from build123d import *

# Parameters (mm, degrees)
F0_W          = 20
F0_H          = 26
F1_DEPTH      = 28
F3_DEPTH      = 3.25
F3_DEPTH_BACK = 3.25
F4_T1_DEPTH   = 6.3508529611
F4_T3_DEPTH   = 6.3508529611
F4_T5_DEPTH   = 6.3508529611
F4_T7_DEPTH   = 6.3508529611
F4_T9_DEPTH   = 51.7168298797
F4_T11_DEPTH  = 45.7168298797
F4_T13_DEPTH  = 53.7168298797
F4_T15_DEPTH  = 32.4668298797
F4_T17_DEPTH  = 32.4668298797


# Not quite as in the source:
# - a fillet or chamfer that OpenCascade refuses, or shapes differently, is made with other operations: its cross-section is extruded or revolved along the edge and cut away or added


with BuildPart() as f1:
    # F0 (on Top) → F1 (new body)
    with BuildSketch(Plane.XY):
        Rectangle(F0_W, F0_H)
    extrude(amount=F1_DEPTH)

    # F2 (on Right) → F3 (cut, two sides)
    with BuildSketch(Plane.YZ) as f3_sk:
        Polygon((13, 28), (-11, 28), (-11, 19.4068542495), (-5.3431457505, 13.75), (13, 13.75), align=None)
    extrude(amount=-F3_DEPTH, mode=Mode.SUBTRACT)
    extrude(f3_sk.sketch, amount=F3_DEPTH_BACK, mode=Mode.SUBTRACT)

    # F4: chamfer of 5 on 9 edges, made by hand

    # F4_s2 → F4_t1 (cut)
    with BuildSketch(Plane(origin=(13.6666666667, -13.6666666667, 13.6666666667), x_dir=(0.7071067812, 0.7071067812, 0), z_dir=(0.5773502692, -0.5773502692, 0.5773502692))):
        Polygon((1.4142135624, 11.430952133), (-5.6568542495, 11.430952133), (-2.1213203436, 17.5546764899), align=None)
    extrude(amount=F4_T1_DEPTH, mode=Mode.SUBTRACT)

    # F4_s4 → F4_t3 (cut)
    with BuildSketch(Plane(origin=(13.6666666667, 13.6666666667, 13.6666666667), x_dir=(-0.7071067812, 0.7071067812, 0), z_dir=(0.5773502692, 0.5773502692, 0.5773502692))):
        Polygon((-1.4142135624, 11.430952133), (5.6568542495, 11.430952133), (2.1213203436, 17.5546764899), align=None)
    extrude(amount=F4_T3_DEPTH, mode=Mode.SUBTRACT)

    # F4_s6 → F4_t5 (cut)
    with BuildSketch(Plane(origin=(-13.6666666667, -13.6666666667, 13.6666666667), x_dir=(0.7071067812, -0.7071067812, 0), z_dir=(-0.5773502692, -0.5773502692, 0.5773502692))):
        Polygon((5.6568542495, 11.430952133), (2.1213203436, 17.5546764899), (-1.4142135624, 11.430952133), align=None)
    extrude(amount=F4_T5_DEPTH, mode=Mode.SUBTRACT)

    # F4_s8 → F4_t7 (cut)
    with BuildSketch(Plane(origin=(-13.6666666667, 13.6666666667, 13.6666666667), x_dir=(-0.7071067812, -0.7071067812, 0), z_dir=(-0.5773502692, 0.5773502692, 0.5773502692))):
        Polygon((-5.6568542495, 11.430952133), (-2.1213203436, 17.5546764899), (1.4142135624, 11.430952133), align=None)
    extrude(amount=F4_T7_DEPTH, mode=Mode.SUBTRACT)

    # F4_s10 → F4_t9 (cut)
    with BuildSketch(Plane.XZ.offset(-25.8584149398)):
        Polygon((10, 23), (5, 28), (10, 28), align=None)
        Polygon((-5, 28), (-10, 23), (-10, 28), align=None)
    extrude(amount=F4_T9_DEPTH, mode=Mode.SUBTRACT)

    # F4_s12 → F4_t11 (cut)
    with BuildSketch(Plane.YZ.offset(-22.8584149398)):
        Polygon((-13, 23), (-8, 28), (-13, 28), align=None)
    extrude(amount=F4_T11_DEPTH, mode=Mode.SUBTRACT)

    # F4_s14 → F4_t13 (cut)
    with BuildSketch(Plane.XY.offset(-12.8584149398)):
        Polygon((10, -8), (5, -13), (10, -13), align=None)
        Polygon((-5, -13), (-10, -8), (-10, -13), align=None)
        Polygon((10, 8), (5, 13), (10, 13), align=None)
        Polygon((-5, 13), (-10, 8), (-10, 13), align=None)
    extrude(amount=F4_T13_DEPTH, mode=Mode.SUBTRACT)

    # F4_s16 → F4_t15 (cut)
    with BuildSketch(Plane.YZ.offset(-22.8584149398)):
        Polygon((13, 23), (8, 28), (13, 28), align=None)
    extrude(amount=F4_T15_DEPTH, mode=Mode.SUBTRACT)

    # F4_s18 → F4_t17 (cut)
    with BuildSketch(Plane.YZ.offset(-9.6084149398)):
        Polygon((13, 23), (8, 28), (13, 28), align=None)
    extrude(amount=F4_T17_DEPTH, mode=Mode.SUBTRACT)


solid = f1.part
Geometry check sheet. Reference: the model listing, model coordinates, mm. A direction names the side the tool comes from. Give positions to 0.01 mm unless a question says otherwise; leave off trailing zeros. Order: outer loops, then holes, each group sorted by start corner. A loop starts at its lowest first (then second) coordinate and runs counter-clockwise, first axis right, second up.
1) Tool access check on faces 4 (the flat face through (7, -9, 25)), 5 (the flat face through (3.25, 1, 21)). Record the directions out of +Z, -Z, +X, -X, +Y, -Y that give a thin tool (end or side, any length) a straight path to the whole face; none if there is none.
Results are:
face 4: +Z, +X, -Y
face 5: +Z, +Y
2) Cross-section at D-D (z = 20). Record the boundary of the cut face in (x, y), then the cut area to 3 significant figures.
Results are:
outline: (-10, -8) - (-5, -13) - (5, -13) - (10, -8) - (10, 8) - (5, 13) - (3.25, 13) - (3.25, -11) - (-3.25, -11) - (-3.25, 13) - (-5, 13) - (-10, 8) - close
area: 314 mm2
3) Cross-section at C-C (y = -4.25). Record the boundary of the cut face in (x, z).
Results are:
outline: (-10, 0) - (10, 0) - (10, 23) - (5, 28) - (3.25, 28) - (3.25, 13.75) - (-3.25, 13.75) - (-3.25, 28) - (-5, 28) - (-10, 23) - close
4) Cross-section at B-B (z = 10). Record the boundary of the cut face in (x, y), then the cut area to 3 significant figures.
Results are:
outline: (-10, -8) - (-5, -13) - (5, -13) - (10, -8) - (10, 8) - (5, 13) - (-5, 13) - (-10, 8) - close
area: 470 mm2
5) Gauge pin test, flat end, axial feed: pin 1 (1.7 mm diameter, centred on x = 1.5, z = 23.5, fed in from +Y). Record the tip position at first contact, or that the pin passes through.
Results are:
pin 1: stops at y = -11
6) Draft check along X on faces 1 (the flat face through (-7, 9, 25)), 2 (the flat face through (0, -11, 22)), 3 (the flat face through (10, 0, 11)). Enter one of: released by +X, released by -X, zero draft, split by the parting line, or undercut.
Results are:
face 1: released by -X
face 2: undercut
face 3: released by +X
7) Material ranges on probe 1 along X at (y, z) = (0.5, 14.25); probe 2 along Y at (x, z) = (2, 22); probe 3 along Z at (x, y) = (1, 0), recorded low to high.
Results are:
probe 1: x = -10 to -3.25, 3.25 to 10
probe 2: y = -13 to -11
probe 3: z = 0 to 13.75
8) Cross-section at A-A (x = -1). Record the boundary of the cut face in (y, z), then the cut area to 3 significant figures.
Results are:
outline: (-13, 0) - (13, 0) - (13, 13.75) - (-5.34, 13.75) - (-11, 19.41) - (-11, 25) - (-13, 23) - close
area: 394 mm2
